Geometry: final body of the model. Coordinates: model frame, mm. Face numbers are marked on the shaded views. A direction names the side the tool comes from. Coordinates: 2 decimals unless noted, no trailing zeros. Write each loop counter-clockwise with the first axis right and the second up, starting at its lowest first coordinate (ties: lowest second). Pieces come first, ordered by that corner, then holes.
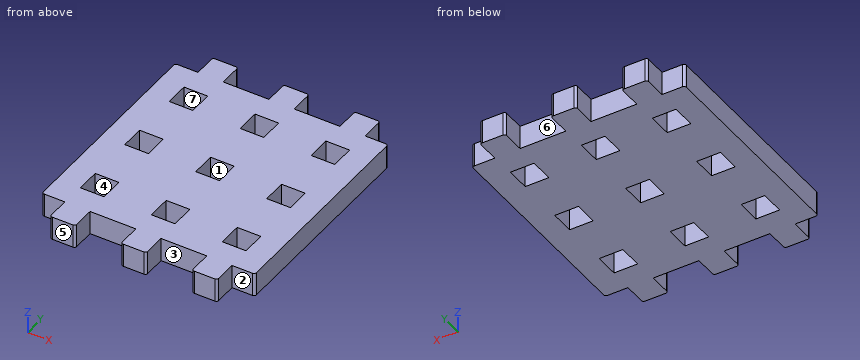
from build123d import *

# Parameters (mm, degrees)
MODEL_W                 = 3
MODEL_H                 = 3
MODEL_W_2               = 3.000000001
SALIENTE_EXTRUIR1_DEPTH = 3


with BuildPart() as part:
    # Model → Saliente-Extruir1 (new body)
    with BuildSketch(Plane.XY):
        with BuildLine():
            Line((8.96548528, 297.776664772), (8.96548528, 271.376664772))
            ThreePointArc((8.96548528, 271.376664772), (9.053353246, 271.164532738), (9.265485281, 271.076664772))
            Line((9.265485281, 271.076664772), (11.86548528, 271.076664772))
            Line((11.86548528, 271.076664772), (11.86548528, 268.376664772))
            ThreePointArc((11.86548528, 268.376664772), (11.953353246, 268.164532738), (12.165485281, 268.076664772))
            Line((12.165485281, 268.076664772), (14.765485281, 268.076664772))
            ThreePointArc((14.765485281, 268.076664772), (14.977617315, 268.164532738), (15.065485281, 268.376664772))
            Line((15.065485281, 268.376664772), (15.065485281, 271.076664772))
            Line((15.065485281, 271.076664772), (20.86548528, 271.076664772))
            Line((20.86548528, 271.076664772), (20.86548528, 268.376664772))
            ThreePointArc((20.86548528, 268.376664772), (20.953353246, 268.164532738), (21.165485281, 268.076664772))
            Line((21.165485281, 268.076664772), (23.76548528, 268.076664772))
            ThreePointArc((23.76548528, 268.076664772), (23.977617315, 268.164532738), (24.06548528, 268.376664772))
            Line((24.06548528, 268.376664772), (24.06548528, 271.076664772))
            Line((24.06548528, 271.076664772), (29.86548528, 271.076664772))
            Line((29.86548528, 271.076664772), (29.86548528, 268.376664772))
            ThreePointArc((29.86548528, 268.376664772), (29.953353246, 268.164532738), (30.165485281, 268.076664772))
            Line((30.165485281, 268.076664772), (32.765485281, 268.076664772))
            ThreePointArc((32.765485281, 268.076664772), (32.977617315, 268.164532738), (33.06548528, 268.376664772))
            Line((33.06548528, 268.376664772), (33.06548528, 271.076664772))
            Line((33.06548528, 271.076664772), (35.66548528, 271.076664772))
            ThreePointArc((35.66548528, 271.076664772), (35.877617315, 271.164532738), (35.96548528, 271.376664772))
            Line((35.96548528, 271.376664772), (35.96548528, 297.776664772))
            ThreePointArc((35.96548528, 297.776664772), (35.877617315, 297.988796806), (35.66548528, 298.076664772))
            Line((35.66548528, 298.076664772), (33.06548528, 298.076664772))
            Line((33.06548528, 298.076664772), (33.06548528, 300.776664772))
            ThreePointArc((33.06548528, 300.776664772), (32.977617315, 300.988796806), (32.765485281, 301.076664772))
            Line((32.765485281, 301.076664772), (30.165485281, 301.076664772))
            ThreePointArc((30.165485281, 301.076664772), (29.953353246, 300.988796806), (29.86548528, 300.776664772))
            Line((29.86548528, 300.776664772), (29.86548528, 298.076664772))
            Line((29.86548528, 298.076664772), (24.06548528, 298.076664772))
            Line((24.06548528, 298.076664772), (24.06548528, 300.776664772))
            ThreePointArc((24.06548528, 300.776664772), (23.977617315, 300.988796806), (23.76548528, 301.076664772))
            Line((23.76548528, 301.076664772), (21.165485281, 301.076664772))
            ThreePointArc((21.165485281, 301.076664772), (20.953353246, 300.988796806), (20.86548528, 300.776664772))
            Line((20.86548528, 300.776664772), (20.86548528, 298.076664772))
            Line((20.86548528, 298.076664772), (15.065485281, 298.076664772))
            Line((15.065485281, 298.076664772), (15.065485281, 300.776664772))
            ThreePointArc((15.065485281, 300.776664772), (14.977617315, 300.988796806), (14.765485281, 301.076664772))
            Line((14.765485281, 301.076664772), (12.165485281, 301.076664772))
            ThreePointArc((12.165485281, 301.076664772), (11.953353246, 300.988796806), (11.86548528, 300.776664772))
            Line((11.86548528, 300.776664772), (11.86548528, 298.076664772))
            Line((11.86548528, 298.076664772), (9.265485281, 298.076664772))
            ThreePointArc((9.265485281, 298.076664772), (9.053353246, 297.988796806), (8.96548528, 297.776664772))
        make_face()
        with Locations((13.46548528, 293.576664772)):
            Rectangle(MODEL_W, MODEL_H, mode=Mode.SUBTRACT)
        with Locations((22.465485281, 293.576664772)):
            Rectangle(MODEL_W_2, MODEL_H, mode=Mode.SUBTRACT)
        with Locations((31.46548528, 293.576664772)):
            Rectangle(MODEL_W, MODEL_H, mode=Mode.SUBTRACT)
        with Locations((13.46548528, 275.576664772)):
            Rectangle(MODEL_W, MODEL_H, mode=Mode.SUBTRACT)
        with Locations((22.465485281, 275.576664772)):
            Rectangle(MODEL_W_2, MODEL_H, mode=Mode.SUBTRACT)
        with Locations((31.46548528, 275.576664772)):
            Rectangle(MODEL_W, MODEL_H, mode=Mode.SUBTRACT)
        with Locations((13.46548528, 284.576664772)):
            Rectangle(MODEL_W, MODEL_H, mode=Mode.SUBTRACT)
        with Locations((22.465485281, 284.576664772)):
            Rectangle(MODEL_W_2, MODEL_H, mode=Mode.SUBTRACT)
        with Locations((31.46548528, 284.576664772)):
            Rectangle(MODEL_W, MODEL_H, mode=Mode.SUBTRACT)
    extrude(amount=SALIENTE_EXTRUIR1_DEPTH)


solid = part.part
Item 1: Section D-D, the plane x = 16.75. Output: boundary loops of the cut face in (y, z).
Derived:
outline: (271.08, 0) - (298.08, 0) - (298.08, 3) - (271.08, 3) - close
Item 2: Section C-C, the plane z = 0.4. State how many separate pieces and enclosed holes the cut face has, plus the area to 3 significant figures.
Derived:
separate pieces: 1
enclosed holes: 9
area: 705 mm2
Item 3: Section A-A, the plane y = 276. Output: boundary loops of the cut face in (x, z), plus the area to 3 significant figures.
Derived:
outline: (8.97, 0) - (11.97, 0) - (11.97, 3) - (8.97, 3) - close; (14.97, 0) - (20.97, 0) - (20.97, 3) - (14.97, 3) - close; (23.97, 0) - (29.97, 0) - (29.97, 3) - (23.97, 3) - close; (32.97, 0) - (35.97, 0) - (35.97, 3) - (32.97, 3) - close
area: 54.0 mm2
Item 4: Material intervals for probe 1 along X at (y, z) = (293, 1.7); probe 2 along Y at (x, z) = (13.5, 2.45); probe 3 along X at (y, z) = (299, 1.3), sorted ascending.
Derived:
probe 1: x = 8.97 to 11.97, 14.97 to 20.97, 23.97 to 29.97, 32.97 to 35.97
probe 2: y = 268.08 to 274.08, 277.08 to 283.08, 286.08 to 292.08, 295.08 to 301.08
probe 3: x = 11.87 to 15.07, 20.87 to 24.07, 29.87 to 33.07
Item 5: Pin query (flat end, axial travel): pin 1 (1.3 mm diameter, centred on x = 34.5, z = 1.5, fed in from +Y). Return the tip coordinate at first contact, or that it passes through.
Derived:
pin 1: stops at y = 298.08
Item 6: Set-up query: the marked faces 1, 2 and 3. Return all of +Z, -Z, +X, -X, +Y, -Y with unobstructed straight access to the full face (end or side cutting, diameter ignored); none if empty.
Derived:
face 1: +Z, -Z
face 2: +Z, -Z, +X, -Y
face 3: +Z, -Z, -Y
Item 7: Section B-B, the plane x = 31. Output: boundary loops of the cut face in (y, z), plus the area to 3 significant figures.
Derived:
outline: (268.08, 0) - (274.08, 0) - (274.08, 3) - (268.08, 3) - close; (277.08, 0) - (283.08, 0) - (283.08, 3) - (277.08, 3) - close; (286.08, 0) - (292.08, 0) - (292.08, 3) - (286.08, 3) - close; (295.08, 0) - (301.08, 0) - (301.08, 3) - (295.08, 3) - close
area: 72.0 mm2
Item 8: Pull-direction query (Y, two-part tool) for the marked faces 4, 5, 6 and 7; classes: released by +Y, released by -Y, zero draft, split by the parting line, or undercut.
Derived:
face 4: undercut
face 5: released by -Y
face 6: released by +Y
face 7: undercut
